Verification items for this drawing (mm, ordinates from the low corner). Coordinates: 2 decimals unless noted, no trailing zeros. Loops run counter-clockwise (first coordinate to the right, second up) from the corner with the lowest first, then second, coordinate; pieces in that order, holes last.
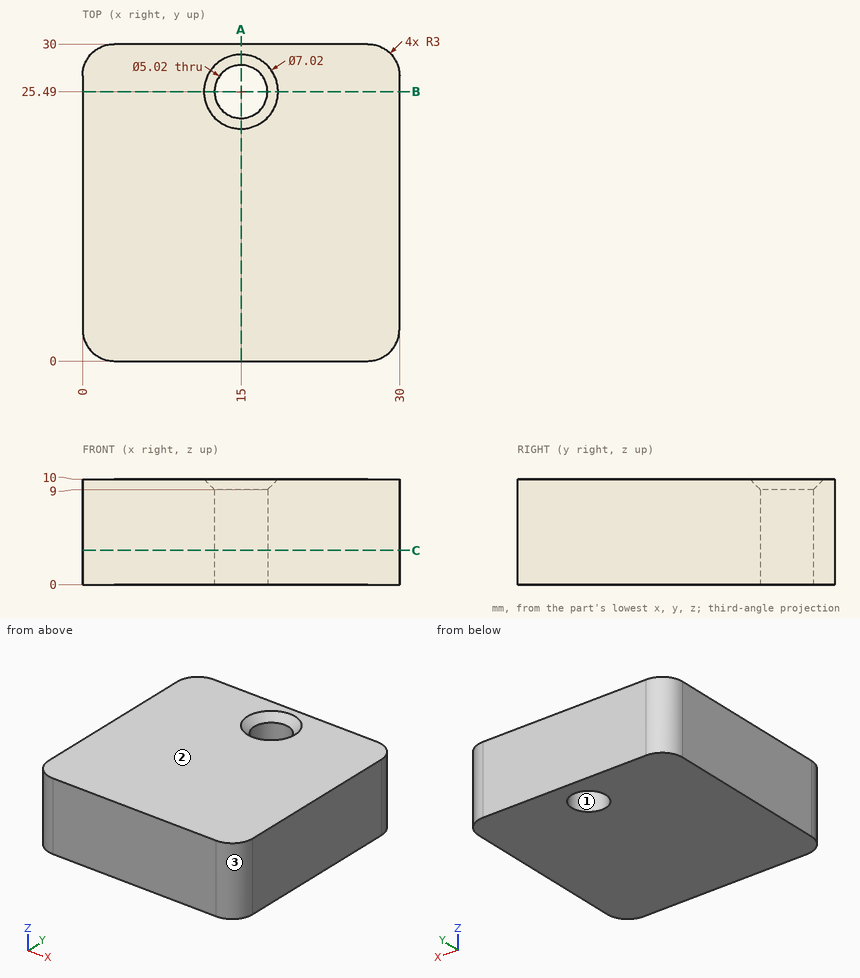
(1) Section check A-A, the plane x = 15. Enter the section's corners in (y, z).
(2) Scan lines: line 1 along Y through (x, z) = (15, 5.75); line 2 along Y through (x, z) = (17.25, 6.5); line 3 along X through (y, z) = (27.75, 3.5). Record each from-to range of solid material in increasing order.
(3) Section check B-B, the plane y = 25.49. Enter the section's corners in (x, z).
(4) Draft check along Y on the marked faces 1, 2 and 3. Enter one of: pulls with the +Y half, pulls with the -Y half, needs draft (parallel to the pull), parting line crosses it, or undercut.
(5) Section check C-C, the plane z = 3.25. Enter the section's corners in (x, y), plus the area to 3 significant figures.
Determined:
1. outline: (0, 0) - (22.98, 0) - (22.98, 9) - (21.98, 10) - (0, 10) - close; (28, 0) - (30, 0) - (30, 10) - (29, 10) - (28, 9) - close
2. line 1: y = 0 to 22.98, 28 to 30
2. line 2: y = 0 to 24.38, 26.6 to 30
2. line 3: x = 0.1 to 13.91, 16.09 to 29.9
3. outline: (0, 0) - (12.49, 0) - (12.49, 9) - (11.49, 10) - (0, 10) - close; (17.51, 0) - (30, 0) - (30, 10) - (18.51, 10) - (17.51, 9) - close
4. face 1: undercut
4. face 2: needs draft
4. face 3: pulls with the -Y half
5. outline: (0, 3) arc R3 ccw to (3, 0) - (27, 0) arc R3 ccw to (30, 3) - (30, 27) arc R3 ccw to (27, 30) - (3, 30) arc R3 ccw to (0, 27) - close; hole circle Ø5.02 at (15, 25.49)
5. area: 872 mm2
